```python
from build123d import *

# Parameters (mm, degrees)
SKETCH1_W          = 50.8
SKETCH1_H          = 50.8
SKETCH1_R          = 6.35
SKETCH1_R_2        = 3.2639
EXTRUDE1_DEPTH     = 12.7
SKETCH2_R          = 5.1562
CUT_EXTRUDE1_DEPTH = 6.604
CHAMFER1_SIZE      = 0.254


with BuildPart() as part:
    # Sketch1 → Extrude1 (new body)
    with BuildSketch(Plane(origin=(0, 0, 0), x_dir=(1, 0, 0), z_dir=(0, 1, 0))):
        with Locations((-25.4, 25.4)):
            Rectangle(SKETCH1_W, SKETCH1_H)
        with Locations(Location((-38.1, 38.1, 0), (0, 0, 270))):
            Circle(SKETCH1_R, mode=Mode.SUBTRACT)
        with Locations(Location((-12.7, 38.1, 0), (0, 0, 270))):
            Circle(SKETCH1_R_2, mode=Mode.SUBTRACT)
        with Locations(Location((-12.7, 12.7, 0), (0, 0, 270))):
            Circle(SKETCH1_R_2, mode=Mode.SUBTRACT)
        with Locations(Location((-38.1, 12.7, 0), (0, 0, 270))):
            Circle(SKETCH1_R_2, mode=Mode.SUBTRACT)
    extrude(amount=EXTRUDE1_DEPTH)

    # Sketch2 → Cut-Extrude1 (cut)
    with BuildSketch(Plane(origin=(0, 12.7, 0), x_dir=(1, 0, 0), z_dir=(0, 1, 0))):
        with Locations(Location((-12.7, 38.1, 0), (0, 0, 270))):
            Circle(SKETCH2_R)
        with Locations(Location((-12.7, 12.7, 0), (0, 0, 270))):
            Circle(SKETCH2_R)
        with Locations(Location((-38.1, 12.7, 0), (0, 0, 270))):
            Circle(SKETCH2_R)
    extrude(amount=-CUT_EXTRUDE1_DEPTH, mode=Mode.SUBTRACT)

    # Chamfer1
    chamfer1_edges = [part.edges().sort_by_distance(p)[0] for p in [
        (-50.8, 12.7, -25.4),
        (-25.4, 12.7, 0),
        (0, 12.7, -25.4),
        (-25.4, 0, 0),
        (-50.8, 0, -25.4),
        (-25.4, 0, -50.8),
        (0, 0, -25.4),
        (-25.4, 12.7, -50.8),
        (0, 6.35, 0),
        (-50.8, 6.35, 0),
        (-50.8, 6.35, -50.8),
        (0, 6.35, -50.8),
    ]]
    chamfer(chamfer1_edges, length=CHAMFER1_SIZE)


solid = part.part
```
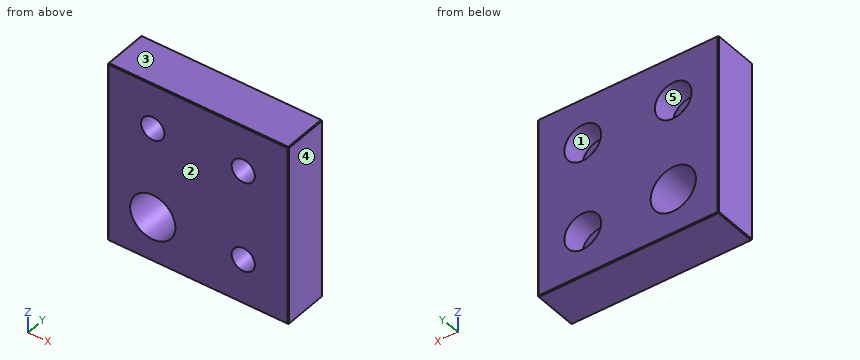
Work out the finished part from the listing and answer in its coordinate system (mm). Face numbers are marked on the shaded views. A direction names the side the tool comes from. Round coordinates to 2 decimals unless told otherwise and drop trailing zeros. Write each loop counter-clockwise with the first axis right and the second up, starting at its lowest first coordinate (ties: lowest second). Pieces come first, ordered by that corner, then holes. Notation, with made-up numbers: (-35, 2.25) - (-28, 2.25) arc R15 ccw to (-28, 17.25) - close; hole circle Ø10 at (8, 2). An arc over 180 degrees is marked (long way). Return JSON: item names as keys, results as strings. Group by question number.
Q1. The mould has two halves that part along X. Classify the marked faces 3, 4 and 5: released by +X, released by -X, zero draft, split by the parting line, or undercut.
Q2. The part is cut by section C-C on x = -38.1. Write down the section's boundary in (y, z).
Q3. Find the intervals of material crossed by L1, parallel to Z at x = -12.7, y = 2.25; L2, parallel to X at y = 10, z = -12.7, in increasing order.
Q4. The part is cut by section D-D on z = -42.5. Write down the section's boundary in (x, y), then the cut area to 3 significant figures.
Q5. The part is cut by section B-B on y = 10.75. Write down the section's boundary in (x, z).
Q6. This flat-tipped pin is pushed along its axis until it touches: pin 1 Ø5 at (x, z) = (-13.5, -14) entering from +Y. Where does it stop, or does it pass through?
Q7. For the marked faces 1 and 2, determine the directions among +Z, -Z, +X, -X, +Y, -Y from which every point of the face is accessible in a straight line to the end or side of a thin tool.
Q8. The part is cut by section A-A on z = -12.7. Write down the section's boundary in (x, y), then the cut area to 3 significant figures.
Solved:
{
 "1": {"face 3": "zero draft", "face 4": "released by +X", "face 5": "undercut"},
 "2": {"outline": "(0, -50.55) - (0.25, -50.8) - (12.45, -50.8) - (12.7, -50.55) - (12.7, -44.45) - (0, -44.45) - close; (0, -31.75) - (12.7, -31.75) - (12.7, -17.86) - (6.1, -17.86) - (6.1, -15.96) - (0, -15.96) - close; (0, -9.44) - (6.1, -9.44) - (6.1, -7.54) - (12.7, -7.54) - (12.7, -0.25) - (12.45, 0) - (0.25, 0) - (0, -0.25) - close"},
 "3": {"L1": "-50.8 to -41.36, -34.84 to -15.96, -9.44 to 0", "L2": "-50.8 to -43.26, -32.94 to -17.86, -7.54 to 0"},
 "4": {"outline": "(-50.8, 0.25) - (-50.55, 0) - (-42.68, 0) - (-42.68, 12.7) - (-50.55, 12.7) - (-50.8, 12.45) - close; (-33.52, 0) - (-0.25, 0) - (0, 0.25) - (0, 12.45) - (-0.25, 12.7) - (-10.01, 12.7) - (-10.01, 6.1) - (-15.39, 6.1) - (-15.39, 12.7) - (-33.52, 12.7) - close", "area": "493 mm²"},
 "5": {"outline": "(-50.8, -50.55) - (-50.55, -50.8) - (-0.25, -50.8) - (0, -50.55) - (0, -0.25) - (-0.25, 0) - (-50.55, 0) - (-50.8, -0.25) - close; hole circle Ø12.7 at (-38.1, -38.1); hole circle Ø10.31 at (-38.1, -12.7); hole circle Ø10.31 at (-12.7, -38.1); hole circle Ø10.31 at (-12.7, -12.7)"},
 "6": {"pin 1": "y = 6.1"},
 "7": {"face 1": "+Y", "face 2": "+Z, -Z, +X, -X, -Y"},
 "8": {"outline": "(-50.8, 0.25) - (-50.55, 0) - (-41.36, 0) - (-41.36, 6.1) - (-43.26, 6.1) - (-43.26, 12.7) - (-50.55, 12.7) - (-50.8, 12.45) - close; (-34.84, 0) - (-15.96, 0) - (-15.96, 6.1) - (-17.86, 6.1) - (-17.86, 12.7) - (-32.94, 12.7) - (-32.94, 6.1) - (-34.84, 6.1) - close; (-9.44, 0) - (-0.25, 0) - (0, 0.25) - (0, 12.45) - (-0.25, 12.7) - (-7.54, 12.7) - (-7.54, 6.1) - (-9.44, 6.1) - close", "area": "429 mm²"}
}
